```python
from build123d import *

# Parameters (mm, degrees)
SKETCH1_R           = 1.75
BOSS_EXTRUDE1_DEPTH = 7
SKETCH_1_R          = 3.6
CUT_EXTRUDE_1_DEPTH = 30.45578681


with BuildPart() as part:
    # Sketch1 → Boss-Extrude1 (new body)
    with BuildSketch(Plane(origin=(0, 4, 0), x_dir=(1, 0, 0), z_dir=(0, 1, 0))):
        with BuildLine():
            Line((1.305695063, -4), (20.643657446, -4))
            ThreePointArc((20.643657446, -4), (24.643657446, 0), (20.643657446, 4))
            Line((20.643657446, 4), (2.081641936, 4))
            ThreePointArc((2.081641936, 4), (2.861028333, 4.588201733), (3.521749436, 5.30713988))
            ThreePointArc((3.521749436, 5.30713988), (3.405395609, 5.596745198), (3.282888305, 5.883801663))
            ThreePointArc((3.282888305, 5.883801663), (1.93527598, 5.894040025), (0.627094961, 5.57027124))
            ThreePointArc((0.627094961, 5.57027124), (0.366286148, 6.046375), (0.084372603, 6.510293938))
            ThreePointArc((0.084372603, 6.510293938), (1.018855105, 7.48132754), (1.683794586, 8.65351323))
            ThreePointArc((1.683794586, 8.65351323), (1.496450048, 8.903135899), (1.303821399, 9.148703928))
            ThreePointArc((1.303821399, 9.148703928), (-0.000522033, 8.809805691), (-1.180330337, 8.158486898))
            ThreePointArc((-1.180330337, 8.158486898), (-1.555477026, 8.550865528), (-1.947855656, 8.926012217))
            ThreePointArc((-1.947855656, 8.926012217), (-1.296536862, 10.105820521), (-0.957638625, 11.410163953))
            ThreePointArc((-0.957638625, 11.410163953), (-1.203206655, 11.602792602), (-1.452829324, 11.79013714))
            ThreePointArc((-1.452829324, 11.79013714), (-2.625015014, 11.125197659), (-3.596048616, 10.190715157))
            ThreePointArc((-3.596048616, 10.190715157), (-4.059967554, 10.472628702), (-4.536071314, 10.733437515))
            ThreePointArc((-4.536071314, 10.733437515), (-4.212302529, 12.041618533), (-4.222540891, 13.389230859))
            ThreePointArc((-4.222540891, 13.389230859), (-4.509597355, 13.511738163), (-4.799202674, 13.62809199))
            ThreePointArc((-4.799202674, 13.62809199), (-5.759348103, 12.682425791), (-6.455432668, 11.528463019))
            ThreePointArc((-6.455432668, 11.528463019), (-6.976508546, 11.680699536), (-7.503891752, 11.809396783))
            ThreePointArc((-7.503891752, 11.809396783), (-7.529737283, 13.156800143), (-7.888414517, 14.455843809))
            ThreePointArc((-7.888414517, 14.455843809), (-8.197396993, 14.499881098), (-8.507248835, 14.537314892))
            ThreePointArc((-8.507248835, 14.537314892), (-9.18992168, 13.375367565), (-9.563620196, 12.080565177))
            ThreePointArc((-9.563620196, 12.080565177), (-10.106342554, 12.09275), (-10.649064912, 12.080565177))
            ThreePointArc((-10.649064912, 12.080565177), (-11.022763428, 13.375367565), (-11.705436272, 14.537314892))
            ThreePointArc((-11.705436272, 14.537314892), (-12.015288115, 14.499881098), (-12.324270591, 14.455843809))
            ThreePointArc((-12.324270591, 14.455843809), (-12.682947825, 13.156800143), (-12.708793355, 11.809396783))
            ThreePointArc((-12.708793355, 11.809396783), (-13.236176561, 11.680699536), (-13.757252439, 11.528463019))
            ThreePointArc((-13.757252439, 11.528463019), (-14.453337005, 12.682425791), (-15.413482434, 13.62809199))
            ThreePointArc((-15.413482434, 13.62809199), (-15.703087752, 13.511738163), (-15.990144217, 13.389230859))
            ThreePointArc((-15.990144217, 13.389230859), (-16.000382579, 12.041618533), (-15.676613793, 10.733437515))
            ThreePointArc((-15.676613793, 10.733437515), (-16.152717554, 10.472628702), (-16.616636492, 10.190715157))
            ThreePointArc((-16.616636492, 10.190715157), (-17.587670094, 11.125197659), (-18.759855783, 11.79013714))
            ThreePointArc((-18.759855783, 11.79013714), (-19.009478453, 11.602792602), (-19.255046482, 11.410163953))
            ThreePointArc((-19.255046482, 11.410163953), (-18.916148245, 10.105820521), (-18.264829452, 8.926012217))
            ThreePointArc((-18.264829452, 8.926012217), (-18.657208082, 8.550865528), (-19.032354771, 8.158486898))
            ThreePointArc((-19.032354771, 8.158486898), (-20.212163074, 8.809805691), (-21.516506507, 9.148703928))
            ThreePointArc((-21.516506507, 9.148703928), (-21.709135156, 8.903135899), (-21.896479694, 8.65351323))
            ThreePointArc((-21.896479694, 8.65351323), (-21.231540213, 7.48132754), (-20.297057711, 6.510293938))
            ThreePointArc((-20.297057711, 6.510293938), (-20.578971255, 6.046375), (-20.839780068, 5.57027124))
            ThreePointArc((-20.839780068, 5.57027124), (-22.147961087, 5.894040025), (-23.495573413, 5.883801663))
            ThreePointArc((-23.495573413, 5.883801663), (-23.618080717, 5.596745198), (-23.734434544, 5.30713988))
            ThreePointArc((-23.734434544, 5.30713988), (-22.788768345, 4.346994451), (-21.634805572, 3.650909885))
            ThreePointArc((-21.634805572, 3.650909885), (-21.78704209, 3.129834008), (-21.915739337, 2.602450802))
            ThreePointArc((-21.915739337, 2.602450802), (-23.263142697, 2.576605271), (-24.562186363, 2.217928037))
            ThreePointArc((-24.562186363, 2.217928037), (-24.606223651, 1.908945561), (-24.643657446, 1.599093719))
            ThreePointArc((-24.643657446, 1.599093719), (-23.481710119, 0.916420874), (-22.186907731, 0.542722358))
            ThreePointArc((-22.186907731, 0.542722358), (-12.402167869, -11.872817218), (1.305695063, -4))
        make_face()
        with Locations(Location((20.643657446, 0, 0), (0, 0, 90))):
            Circle(SKETCH1_R, mode=Mode.SUBTRACT)
    extrude(amount=-BOSS_EXTRUDE1_DEPTH)

    # 草图1 → 切除-拉伸1 (cut, through all)
    with BuildSketch(Plane.XZ.offset(3)):
        with Locations(Location((-10.106342554, 0, 0), (0, 0, 270))):
            Circle(SKETCH_1_R)
    extrude(amount=-CUT_EXTRUDE_1_DEPTH, mode=Mode.SUBTRACT)


solid = part.part
```
Could you check a few things on this model? Use its own coordinates, in mm. A direction names the side the tool comes from. Give positions to 0.01 mm unless a question says otherwise; leave off trailing zeros. Order: outer loops, then holes, each group sorted by start corner. A loop starts at its lowest first (then second) coordinate and runs counter-clockwise, first axis right, second up.
Q1. Suppose I cut it at B-B, the plane x = 11.5. Write out the boundary of the cut face in (y, z).
Q2. Suppose I cut it at C-C, the plane y = -0.25. Count the separate pieces of the cut face and the enclosed holes in it, and give its area (3 significant figures).
Q3. We'd pull the mould along X, two halves only. Please class faces 1 (the cylindrical face through (-16.146, 0.549, -10.476)), 2 (the cylindrical face through (-22.804, 0.549, -4.359)), 3 (the flat face through (11, 1, 4)): +X half, -X half, draft (parallel to the pull), parting line (faces both ways), or undercut.
Q4. Suppose I cut it at A-A, the plane z = 0. Write out the boundary of the cut face in (x, y).
Q5. If I drill on line 1 along X through (y, z) = (2.5, 0); line 2 along Z through (x, y) = (-10, 1.75); line 3 along Z through (x, y) = (5.5, 1), over which ranges is the centre line in solid material (lowest first)?
Q6. For faces 4 (the cylindrical face through (-21.243, 0.549, -7.497)), 5 (the cylindrical face through (-4.215, 0.549, -12.023)), 6 (the cylindrical face through (-11.015, 0.549, -13.358)), which set-ups out of +Z, -Z, +X, -X, +Y, -Y let a thin tool reach every point of the face, with its end or its side?
Q7. I'm going to push flat-ended pins straight in: P1, Ø4, axis at x = 20.64, z = 0, coming from the +Y side; P2, Ø2, axis at y = -0.5, z = -10, coming from the -X side; P3, Ø2, axis at x = 8, y = -1, coming from the -Z side; P4, Ø3.5, axis at x = 14.5, y = -0.5, coming from the +Z side. Where does each tip first touch, or does it pass through?
Solution:
1. outline: (-3, -4) - (4, -4) - (4, 4) - (-3, 4) - close
2. separate pieces: 1
2. enclosed holes: 2
2. area: 629 mm2
3. face 1: undercut
3. face 2: -X half
3. face 3: draft
4. outline: (-22.2, -3) - (-13.71, -3) - (-13.71, 4) - (-22.2, 4) - close; (-6.51, -3) - (18.89, -3) - (18.89, 4) - (-6.51, 4) - close; (22.39, -3) - (24.64, -3) - (24.64, 4) - (22.39, 4) - close
5. line 1: x = -22.2 to -13.71, -6.51 to 18.89, 22.39 to 24.64
5. line 2: z = -12.09 to -3.6, 3.6 to 12.09
5. line 3: z = -4 to 4
6. face 4: -X, +Y, -Y
6. face 5: +Y, -Y
6. face 6: -Z, +Y, -Y
7. P1: stops at y = 4
7. P2: stops at x = -21.63
7. P3: stops at z = -4
7. P4: stops at z = 4
